CAD build for the part. Positions are in the model's coordinates, mm. A direction names the side the tool comes from. Coordinates: 2 decimals unless noted, no trailing zeros. Order: outer loops, then holes, each group sorted by start corner. A loop starts at its lowest first (then second) coordinate and runs counter-clockwise, first axis right, second up. Notation, with made-up numbers: M 26.5,-14 L 54.5,-14 A21 ccw 54.5,-1 Z; hole C 47,43 d9. An arc over 180 degrees is marked long. One line per item, written item: value.
from build123d import *

# Parameters (mm, degrees)
F0_W     = 133.2214027643
F0_H     = 112.6486063004
F1_DEPTH = 114.808
F2_W     = 105.6237369776
F2_H     = 94.5846736431
F3_DEPTH = 100.838
F4_W     = 36.8804913014
F4_H     = 24.8378776014
F4_W_2   = 31.8627543747
F4_H_2   = 34.8733980209
F5_DEPTH = 56.388
F6_R     = 9.4091261345
F7_DEPTH = 94.742


with BuildPart() as f1:
    # F0 (on Top) → F1 (new body)
    with BuildSketch(Plane.XY):
        Rectangle(F0_W, F0_H)
    extrude(amount=F1_DEPTH)

    # F2 (on face) → F3 (cut)
    with BuildSketch(Plane.XY.offset(114.808)):
        Rectangle(F2_W, F2_H)
    extrude(amount=-F3_DEPTH, mode=Mode.SUBTRACT)

    # F4 (on face) → F5 (join)
    with BuildSketch(Plane.XY.offset(114.808)):
        with Locations((-34.3716228381, 0)):
            Rectangle(F4_W, F4_H)
        with Locations((34.3716228381, 0)):
            Rectangle(F4_W, F4_H)
        with Locations((0, 29.8556378111)):
            Rectangle(F4_W_2, F4_H_2)
        with Locations((0, -29.8556378111)):
            Rectangle(F4_W_2, F4_H_2)
        Rectangle(F4_W_2, F4_H)
    extrude(amount=-F5_DEPTH)

    # F6 (on face) → F7 (cut)
    with BuildSketch(Plane.XY.offset(114.808)):
        Circle(F6_R)
    extrude(amount=-F7_DEPTH, mode=Mode.SUBTRACT)


solid = f1.part
Q1. Slice it at A-A (z = 24). List the corners of the cut face in (x, y).
Recorded:
outline: M -66.61,-56.32 L 66.61,-56.32 L 66.61,56.32 L -66.61,56.32 Z; hole M -52.81,-47.29 L 52.81,-47.29 L 52.81,47.29 L -52.81,47.29 Z
Q2. Which spindle directions (+Z, -Z, +X, -X, +Y, -Y) get a long thin tool onto all of the face, cutting with end or side? Do faces 5 (the face through (-6.935, 6.359, 87.009)), 6 (the face through (-1, 47.292, 54)), 7 (the face through (-1, -12, 114.808)). Say none if no direction does.
Recorded:
face 5: +Z
face 6: none
face 7: +Z, +X, -X, +Y, -Y
Q3. Mould opens along X. For faces 1 (the face through (-66.611, -1, 57)), 2 (the face through (34, 12.419, 87)), 3 (the face through (-15.931, 30, 87)), 4 (the face through (-1, 1, 0)) say: released by +X, released by -X, zero draft, split by the parting line, or undercut.
Recorded:
face 1: released by -X
face 2: undercut
face 3: undercut
face 4: zero draft
Q4. Drill centre lines: line 1 along X through (y, z) = (-38, 65.5); line 2 along Y through (x, z) = (-49.5, 85); line 3 along Z through (x, y) = (-29.5, 12). Where is each one in solid material? Low to high.
Recorded:
line 1: x = -66.61 to -52.81, -15.93 to 15.93, 52.81 to 66.61
line 2: y = -56.32 to -47.29, -12.42 to 12.42, 47.29 to 56.32
line 3: z = 0 to 13.97, 58.42 to 114.81
Q5. Slice it at B-B (x = 20.5). List the corners of the cut face in (y, z), plus the area to 3 significant figures.
Recorded:
outline: M -56.32,0 L 56.32,0 L 56.32,114.81 L 47.29,114.81 L 47.29,13.97 L -47.29,13.97 L -47.29,114.81 L -56.32,114.81 Z; M -12.42,58.42 L 12.42,58.42 L 12.42,114.81 L -12.42,114.81 Z
area: 4,800 mm^2
Q6. Slice it at D-D (z = 74). List the corners of the cut face in (x, y).
Recorded:
outline: M -66.61,-56.32 L 66.61,-56.32 L 66.61,56.32 L -66.61,56.32 Z; hole M -52.81,-47.29 L -15.93,-47.29 L -15.93,-12.42 L -52.81,-12.42 Z; hole M -52.81,12.42 L -15.93,12.42 L -15.93,47.29 L -52.81,47.29 Z; hole C 0,0 d18.82; hole M 15.93,-47.29 L 52.81,-47.29 L 52.81,-12.42 L 15.93,-12.42 Z; hole M 15.93,12.42 L 52.81,12.42 L 52.81,47.29 L 15.93,47.29 Z
Q7. Pin check, flat tips, straight feed: pin 1 Ø2 at (x, y) = (22.5, 33.5) entering from -Z; pin 2 Ø11.5 at (x, y) = (0, 0) entering from +Z. Stop position of each tip, or through.
Recorded:
pin 1: stops at z = 0
pin 2: stops at z = 13.97
Q8. Slice it at C-C (y = 0). List the corners of the cut face in (x, z).
Recorded:
outline: M -66.61,0 L 66.61,0 L 66.61,114.81 L 9.41,114.81 L 9.41,58.42 L 52.81,58.42 L 52.81,13.97 L -52.81,13.97 L -52.81,58.42 L -9.41,58.42 L -9.41,114.81 L -66.61,114.81 Z
